```python
from build123d import *

# Parameters (mm, degrees)
DUCT_THROAT_START           = 18
SKETCH1_W                   = 60
SKETCH1_H                   = 100
DUCT_THROAT_DEPTH           = 80
CARBON_WALL_SHELL_T         = 2
PIVOT_HOLE_PAIRS_DEPTH      = 218.926593145
PIVOT_HOLE_PAIRS_DEPTH_BACK = 218.926593145
SKETCH2_R                   = 1.5
SKETCH3_R                   = 2.5
SMA_ANCHOR_PEG_DEPTH        = 10
BIAS_ANCHOR_PEG_START       = 10
SKETCH4_R                   = 2.5
BIAS_ANCHOR_PEG_DEPTH       = 10


with BuildPart() as part:
    # Sketch1 → Duct_Throat (new body)
    with BuildSketch(Plane(origin=(0, 0, 0), x_dir=(0, 0, -1), z_dir=(1, 0, 0)).offset(DUCT_THROAT_START)):
        with Locations((0, 140)):
            Rectangle(SKETCH1_W, SKETCH1_H)
    extrude(amount=DUCT_THROAT_DEPTH)

    # Carbon_Wall_Shell
    carbon_wall_shell_openings = [part.faces().sort_by_distance(p)[0] for p in [
        (18, 140, 0),
        (98, 140, 0),
    ]]
    offset(amount=CARBON_WALL_SHELL_T, openings=carbon_wall_shell_openings, kind=Kind.INTERSECTION)

    # Sketch2 → Pivot_Hole_Pairs (cut, two sides: drawn at the far end of the back side and taken through both)
    with BuildSketch(Plane.XY.offset(-PIVOT_HOLE_PAIRS_DEPTH_BACK)):
        with Locations((58, 110)):
            Circle(SKETCH2_R)
        with Locations((58, 130)):
            Circle(SKETCH2_R)
        with Locations((58, 150)):
            Circle(SKETCH2_R)
        with Locations((58, 170)):
            Circle(SKETCH2_R)
    extrude(amount=PIVOT_HOLE_PAIRS_DEPTH + PIVOT_HOLE_PAIRS_DEPTH_BACK, mode=Mode.SUBTRACT)

    # Sketch3 → SMA_Anchor_Peg (add)
    with BuildSketch(Plane(origin=(0, 192, 0), x_dir=(1, 0, 0), z_dir=(0, 1, 0))):
        with Locations(Location((66.342275148, -29, 0), (0, 0, 90))):
            Circle(SKETCH3_R)
    extrude(amount=SMA_ANCHOR_PEG_DEPTH)

    # Sketch4 → Bias_Anchor_Peg (add)
    with BuildSketch(Plane.XZ.offset(-88).offset(BIAS_ANCHOR_PEG_START)):
        with Locations(Location((66.342275148, 29, 0), (0, 0, 270))):
            Circle(SKETCH4_R)
    extrude(amount=-BIAS_ANCHOR_PEG_DEPTH)


solid = part.part
```
Geometry check sheet. Reference: the model listing, model coordinates, mm. A direction names the side the tool comes from. Give positions to 0.01 mm unless a question says otherwise; leave off trailing zeros. Write each loop counter-clockwise with the first axis right and the second up, starting at its lowest first coordinate (ties: lowest second). Pieces come first, ordered by that corner, then holes.
1) Section check C-C, the plane x = 28.5. Record the boundary of the cut face in (y, z).
2) Access from +Z, -Z, +X, -X, +Y, -Y to the whole of each face (thin tool, end or side, straight path). Record for faces 5 (the cylindrical face through (58.806, 131.265, -31.014)), 6 (the flat face through (57, 139, 30)), 7 (the cylindrical face through (68.82, 82.93, 29.33)).
3) Section check A-A, the plane y = 130. Record the boundary of the cut face in (x, z).
4) Section check B-B, the plane z = 14. Record the boundary of the cut face in (x, y), and give its area (3 significant figures).
5) Section check D-D, the plane x = 58. State how many separate pieces and enclosed holes the cut face has, and give its area (3 significant figures).
6) Gauge pin test, flat ends, axial feed: pin 1 (12 mm diameter, centred on x = 79.5, z = -17.5, fed in from -Y); pin 2 (2.5 mm diameter, centred on x = 58, y = 130, fed in from +Z); pin 3 (5 mm diameter, centred on x = 78.5, z = 9, fed in from +Y). Record the tip position at first contact, or that the pin passes through.
7) Material ranges on L1, parallel to Y at x = 58, z = 31; L2, parallel to Z at x = 65, y = 155; L3, parallel to X at y = 110, z = 31.4, recorded low to high.
8) Release check for a two-part mould opening along Z. For faces 1 (the cylindrical face through (68.783, 196.93, 29.542)), 2 (the flat face through (57, 139, -30)), 3 (the cylindrical face through (58.806, 151.265, 30.986)), 4 (the flat face through (57, 139, -32)) record: pulls with the +Z half, pulls with the -Z half, needs draft (parallel to the pull), parting line crosses it, or undercut.
Computed:
1. outline: (88, -32) - (192, -32) - (192, 32) - (88, 32) - close; hole (90, -30) - (190, -30) - (190, 30) - (90, 30) - close
2. face 5: +Z, -Z
2. face 6: +X, -X
2. face 7: -Y
3. outline: (18, -32) - (56.5, -32) - (56.5, -30) - (18, -30) - close; (18, 30) - (56.5, 30) - (56.5, 32) - (18, 32) - close; (59.5, -32) - (98, -32) - (98, -30) - (59.5, -30) - close; (59.5, 30) - (98, 30) - (98, 32) - (59.5, 32) - close
4. outline: (18, 88) - (98, 88) - (98, 90) - (18, 90) - close; (18, 190) - (98, 190) - (98, 192) - (18, 192) - close
4. area: 320 mm2
5. separate pieces: 8
5. enclosed holes: 0
5. area: 608 mm2
6. pin 1: stops at y = 88
6. pin 2: passes through
6. pin 3: stops at y = 192
7. L1: y = 88 to 108.5, 111.5 to 128.5, 131.5 to 148.5, 151.5 to 168.5, 171.5 to 192
7. L2: z = -32 to -30, 30 to 32
7. L3: x = 18 to 56.5, 59.5 to 98
8. face 1: parting line crosses it
8. face 2: undercut
8. face 3: needs draft
8. face 4: pulls with the -Z half
